Part model, mm, in its own coordinate system. A direction names the side the tool comes from. Round coordinates to 2 decimals unless told otherwise and drop trailing zeros. Loops run counter-clockwise (first coordinate to the right, second up) from the corner with the lowest first, then second, coordinate; pieces in that order, holes last. Notation, with made-up numbers: M 6.5,52 L 54.5,52 A24 ccw 54.5,80 Z; hole C -20,-6 d3. An arc over 180 degrees is marked long. Write each question's results on one line, items separated by ' | '.
from build123d import *

# Parameters (mm, degrees)
BOSS_EXTRUDE1_START = -3
SKETCH1_W           = 46
SKETCH1_H           = 44
SKETCH1_R           = 11.5
BOSS_EXTRUDE1_DEPTH = 6
SKETCH3_W           = 46
SKETCH3_H           = 4
BOSS_EXTRUDE2_DEPTH = 16.8
BOSS_EXTRUDE3_DEPTH = 2
BOSS_EXTRUDE4_START = -46
BOSS_EXTRUDE4_DEPTH = 2
SKETCH5_R           = 1.75
CUT_EXTRUDE1_DEPTH  = 42.856535929
SKETCH6_R           = 2.25
CUT_EXTRUDE2_DEPTH  = 55.341880718
FILLET1_R           = 4
FILLET2_START       = -19.0000001
FILLET2_2_DEPTH     = 34.0000001
CHAMFER1_SIZE       = 3


with BuildPart() as part:
    # Sketch1 → Boss-Extrude1 (new body)
    with BuildSketch(Plane(origin=(0, 0, 0), x_dir=(1, 0, 0), z_dir=(0, 1, 0)).offset(BOSS_EXTRUDE1_START)):
        with Locations((-2, -2.64)):
            Rectangle(SKETCH1_W, SKETCH1_H)
        with Locations(Location((-2, -3.64, 0), (0, 0, 270))):
            Circle(SKETCH1_R, mode=Mode.SUBTRACT)
    extrude(amount=BOSS_EXTRUDE1_DEPTH)

    # Sketch3 → Boss-Extrude2 (add)
    with BuildSketch(Plane(origin=(0, 3, 0), x_dir=(1, 0, 0), z_dir=(0, 1, 0))):
        with Locations((-2, 17.36)):
            Rectangle(SKETCH3_W, SKETCH3_H)
    extrude(amount=BOSS_EXTRUDE2_DEPTH)

    # Sketch4 → Boss-Extrude3 (add)
    with BuildSketch(Plane.ZY.offset(25)):
        Polygon((-15.36, 19.8), (-15.36, 3), (24.64, 3), align=None)
    extrude(amount=-BOSS_EXTRUDE3_DEPTH)

    # Sketch4<2> → Boss-Extrude4 (add)
    with BuildSketch(Plane.ZY.offset(25).offset(BOSS_EXTRUDE4_START)):
        Polygon((-15.36, 19.8), (-15.36, 3), (24.64, 3), align=None)
    extrude(amount=BOSS_EXTRUDE4_DEPTH)

    # Sketch5 → Cut-Extrude1 (cut, through all)
    with BuildSketch(Plane.XZ.offset(3)):
        with Locations(Location((-17.273506474, 18.913506474, 0), (0, 0, 270))):
            Circle(SKETCH5_R)
        with Locations(Location((13.273506474, 18.913506474, 0), (0, 0, 270))):
            Circle(SKETCH5_R)
        with Locations(Location((13.273506474, -11.633506474, 0), (0, 0, 270))):
            Circle(SKETCH5_R)
        with Locations(Location((-17.273506474, -11.633506474, 0), (0, 0, 270))):
            Circle(SKETCH5_R)
    extrude(amount=-CUT_EXTRUDE1_DEPTH, mode=Mode.SUBTRACT)

    # Sketch6 → Cut-Extrude2 (cut, through all)
    with BuildSketch(Plane(origin=(0, 0, -19.36), x_dir=(-1, 0, 0), z_dir=(0, 0, -1))):
        with Locations((-9, 13.23890477)):
            Circle(SKETCH6_R)
        with Locations((13, 13.23890477)):
            Circle(SKETCH6_R)
    extrude(amount=-CUT_EXTRUDE2_DEPTH, mode=Mode.SUBTRACT)

    # Fillet1
    # the kernel refuses this fillet: 4 mm, written as the material it adds along each edge
    with BuildSketch(Plane(origin=(-23, 29.8, -15.36), x_dir=(0, 0, 1), z_dir=(0, -1, 0))) as fillet1_piece_1_section:
        with BuildLine():
            CenterArc((FILLET1_R, -FILLET1_R), FILLET1_R, 90, 90)
            Line((0, -FILLET1_R), (0, 0))
            Line((0, 0), (FILLET1_R, 0))
        make_face()
    fillet1_piece_1 = extrude(amount=26.8, mode=Mode.PRIVATE)
    fillet1_piece_1 = split(fillet1_piece_1, bisect_by=Plane(origin=(-23, 21.299489969, -18.930214213), z_dir=(0, -0.9219821056073614, -0.3872324843550918)), keep=Keep.TOP, mode=Mode.PRIVATE)
    add(fillet1_piece_1)
    with BuildSketch(Plane(origin=(19, 29.8, -15.36), x_dir=(0, 0, 1), z_dir=(0, -1, 0))) as fillet1_piece_2_section:
        with BuildLine():
            CenterArc((FILLET1_R, FILLET1_R), FILLET1_R, 180, 90)
            Line((0, FILLET1_R), (0, 0))
            Line((0, 0), (FILLET1_R, 0))
        make_face()
    fillet1_piece_2 = extrude(amount=26.8, mode=Mode.PRIVATE)
    fillet1_piece_2 = split(fillet1_piece_2, bisect_by=Plane(origin=(19, 21.299489969, -18.930214213), z_dir=(0, -0.9219821056073614, -0.3872324843550918)), keep=Keep.TOP, mode=Mode.PRIVATE)
    add(fillet1_piece_2)
    # the kernel refuses this fillet: 4 mm, written as the material it takes off along each edge
    with BuildSketch(Plane(origin=(21, -13, 24.64), x_dir=(-1, 0, 0), z_dir=(0, 1, 0))) as fillet1_2_piece_1:
        with BuildLine():
            CenterArc((FILLET1_R, -FILLET1_R), FILLET1_R, 90, 90)
            Line((0, -FILLET1_R), (0, 0))
            Line((0, 0), (FILLET1_R, 0))
        make_face()
    extrude(amount=26, mode=Mode.SUBTRACT)
    with BuildSketch(Plane(origin=(-25, -13, 24.64), x_dir=(1, 0, 0), z_dir=(0, 1, 0))) as fillet1_2_piece_2:
        with BuildLine():
            CenterArc((FILLET1_R, FILLET1_R), FILLET1_R, 180, 90)
            Line((0, FILLET1_R), (0, 0))
            Line((0, 0), (FILLET1_R, 0))
        make_face()
    extrude(amount=26, mode=Mode.SUBTRACT)

    # Fillet2: read off the stored shape, not the designer's step
    # Fillet2 outline → Fillet2 (revolve, cut)
    with BuildSketch(Plane(origin=(15, 0, -11.36), x_dir=(1, 0, 0), z_dir=(0, 0, 1))):
        with BuildLine():
            ThreePointArc((4, 17.8), (4.585786438, 19.214213562), (6, 19.8))
            Line((6, 19.8), (4, 19.8))
            Line((4, 19.8), (4, 17.8))
        make_face()
    revolve(axis=Axis((15, 0, -11.36), (0, 1, 0)), mode=Mode.SUBTRACT)

    # Fillet2 2 outline → Fillet2 2 (cut)
    with BuildSketch(Plane.YZ.offset(FILLET2_START)):
        with BuildLine():
            Line((19.8, -15.36), (17.8, -15.36))
            ThreePointArc((17.8, -15.36), (19.214213562, -15.945786438), (19.8, -17.36))
            Line((19.8, -17.36), (19.8, -15.36))
        make_face()
    extrude(amount=FILLET2_2_DEPTH, mode=Mode.SUBTRACT)

    # Fillet2 3 outline → Fillet2 3 (revolve, cut)
    with BuildSketch(Plane(origin=(-19, 0, -11.36), x_dir=(1, 0, 0), z_dir=(0, 0, 1))):
        with BuildLine():
            ThreePointArc((4, 17.8), (4.585786438, 19.214213562), (6, 19.8))
            Line((6, 19.8), (4, 19.8))
            Line((4, 19.8), (4, 17.8))
        make_face()
    revolve(axis=Axis((-19, 0, -11.36), (0, 1, 0)), mode=Mode.SUBTRACT)

    # Chamfer1
    chamfer1_edges = [part.edges().sort_by_distance(p)[0] for p in [
        (-2, 3, -7.86),
    ]]
    chamfer(chamfer1_edges, length=CHAMFER1_SIZE)


solid = part.part
Item 1: Band-saw the part on C-C on y = 1.25. Give the cut face in (x, z).
Filled sheet:
outline: M -25,-19.36 L 21,-19.36 L 21,20.64 A4 ccw 17,24.64 L -21,24.64 A4 ccw -25,20.64 Z; hole C -17.27,-11.63 d3.5; hole C -17.27,18.91 d3.5; hole C -2,3.64 d25.5; hole C 13.27,-11.63 d3.5; hole C 13.27,18.91 d3.5
Item 2: Two-plate mould, pull along Z, no slides. Class faces 3 (the flat face through (-2, 8, -19.36)), 4 (the flat face through (-23.832, 11.397, 4.648)), 5 (the flat face through (-23, 9, 2)), 6 (the cylindrical face through (13.799, -0.042, 17.244)): +Z half, -Z half, draft (parallel to the pull), parting line (faces both ways), or undercut.
Filled sheet:
face 3: -Z half | face 4: +Z half | face 5: draft | face 6: undercut
Item 3: Wall check: L1, parallel to X at y = 4.75, z = 12; L2, parallel to X at y = -2.25, z = 3.64; L3, parallel to Z at x = 14, y = -0.75. Give the ranges that are in metal, low to high.
Filled sheet:
L1: -25 to -23, 19 to 21 | L2: -25 to -13.5, 9.5 to 21 | L3: -19.36 to -13.23, -10.04 to 17.32, 20.51 to 24.64
Item 4: Band-saw the part on B-B on y = 14.75. Give the cut face in (x, z).
Filled sheet:
outline: M -25,-19.36 L -14.67,-19.36 L -14.67,-15.36 L -19,-15.36 A4 cw -23,-11.36 L -23,-3.34 L -25,-3.34 Z; M -11.33,-19.36 L 7.33,-19.36 L 7.33,-15.36 L -11.33,-15.36 Z; M 10.67,-19.36 L 21,-19.36 L 21,-3.34 L 19,-3.34 L 19,-11.36 A4 cw 15,-15.36 L 10.67,-15.36 Z
Item 5: Which spindle directions (+Z, -Z, +X, -X, +Y, -Y) get a long thin tool onto all of the face, cutting with end or side? Do faces 1 (the cylindrical face through (-21.859, 10.504, -14.157)), 2 (the cylindrical face through (19.797, -0.067, 23.499)). Say none if no direction does.
Filled sheet:
face 1: +Z, +Y | face 2: +Z, +X, +Y, -Y
Item 6: Drop flat-ended pins along their axis: P1, Ø12, axis at x = 4, z = 16.5, coming from the +Y side; P2, Ø3, axis at x = -17.27, z = -11.63, coming from the +Y side; P3, Ø5.5, axis at x = 13.27, z = 18.91, coming from the -Y side; P4, Ø1, axis at x = 0, y = 15.5, coming from the +Z side. Give the stop position or say it passes through.
Filled sheet:
P1: y = 3 | P2: through | P3: y = -3 | P4: z = -15.36
Item 7: Band-saw the part on D-D on y = 9.25. Give the cut face in (x, z), and give its area (3 significant figures).
Filled sheet:
outline: M -25,-19.36 L 21,-19.36 L 21,9.76 L 19,9.76 L 19,-11.36 A4 cw 15,-15.36 L -19,-15.36 A4 cw -23,-11.36 L -23,9.76 L -25,9.76 Z | area: 291 mm^2
Item 8: Band-saw the part on A-A on x = -2. Give the cut face in (y, z), and give its area (3 significant figures).
Filled sheet:
outline: M -3,-19.36 L 19.8,-19.36 L 19.8,-17.36 A2 ccw 17.8,-15.36 L 3,-15.36 L 3,-10.86 L 0,-7.86 L -3,-7.86 Z; M -3,15.14 L 0,15.14 L 3,18.14 L 3,24.64 L -3,24.64 Z | area: 183 mm^2
